from build123d import *

# Parameters (mm, degrees)
SKETCH1_W           = 50
SKETCH1_H           = 50
SKETCH1_W_2         = 46
SKETCH1_H_2         = 46
BOSS_EXTRUDE1_DEPTH = 10
SKETCH2_W           = 63.639610306
SKETCH2_H           = 63.639610306
SKETCH2_R           = 1.5
BOSS_EXTRUDE2_DEPTH = 3
FILLET2_R           = 5
FILLET3_R           = 2
CHAMFER2_SIZE       = 1


with BuildPart() as part:
    # Sketch1 → Boss-Extrude1 (new body)
    with BuildSketch(Plane(origin=(0, 0, 0), x_dir=(1, 0, 0), z_dir=(0, 1, 0))):
        Rectangle(SKETCH1_W, SKETCH1_H)
        Rectangle(SKETCH1_W_2, SKETCH1_H_2, mode=Mode.SUBTRACT)
    extrude(amount=BOSS_EXTRUDE1_DEPTH)

    # Sketch2 → Boss-Extrude2 (add)
    with BuildSketch(Plane(origin=(0, 10, 0), x_dir=(1, 0, 0), z_dir=(0, 1, 0))):
        Rectangle(SKETCH2_W, SKETCH2_H)
        with Locations(Location((-27.577164466, 27.577164466, 0), (0, 0, 270))):
            Circle(SKETCH2_R, mode=Mode.SUBTRACT)
        with Locations(Location((27.577164466, 27.577164466, 0), (0, 0, 270))):
            Circle(SKETCH2_R, mode=Mode.SUBTRACT)
        with Locations(Location((-27.577164466, -27.577164466, 0), (0, 0, 270))):
            Circle(SKETCH2_R, mode=Mode.SUBTRACT)
        with Locations(Location((27.577164466, -27.577164466, 0), (0, 0, 270))):
            Circle(SKETCH2_R, mode=Mode.SUBTRACT)
        with BuildLine():
            Line((-5, -23), (5, -23))
            Line((5, -23), (5, -18))
            ThreePointArc((5, -18), (0, -13), (-5, -18))
            Line((-5, -18), (-5, -23))
        make_face(mode=Mode.SUBTRACT)
    extrude(amount=BOSS_EXTRUDE2_DEPTH)

    # Fillet2
    fillet2_edges = [part.edges().sort_by_distance(p)[0] for p in [
        (-25, 5, -25),
        (25, 5, -25),
        (25, 5, 25),
        (-25, 5, 25),
    ]]
    fillet(fillet2_edges, radius=FILLET2_R)

    # Fillet3
    fillet3_edges = [part.edges().sort_by_distance(p)[0] for p in [
        (31.819805153, 11.5, 31.819805153),
        (31.819805153, 11.5, -31.819805153),
        (-31.819805153, 11.5, -31.819805153),
        (-31.819805153, 11.5, 31.819805153),
    ]]
    fillet(fillet3_edges, radius=FILLET3_R)

    # Chamfer2
    chamfer2_edges = [part.edges().sort_by_distance(p)[0] for p in [
        (31.234018716, 13, -31.234018716),
        (0, 13, -31.819805153),
        (31.819805153, 13, 0),
        (-31.819805153, 13, 0),
        (0, 13, 31.819805153),
        (31.234018716, 13, 31.234018716),
        (-31.234018716, 13, 31.234018716),
        (-31.234018716, 13, -31.234018716),
    ]]
    chamfer(chamfer2_edges, length=CHAMFER2_SIZE)


solid = part.part
Read the model definition and answer for the solid it produces. Units are mm, in the model's axes. A direction names the side the tool comes from. Give positions to 0.01 mm unless a question says otherwise; leave off trailing zeros. Write each loop counter-clockwise with the first axis right and the second up, starting at its lowest first coordinate (ties: lowest second). Pieces come first, ordered by that corner, then holes. Notation, with made-up numbers: M 23.5,-6.75 L 43.5,-6.75 A35 cw 43.5,25.25 Z; hole C 73,53.25 d2. An arc over 180 degrees is marked long. One line per item, written item: value. Start each with the question number.
(1) Find section D-D (z = -14). Determine the outline of the cut face in (x, y), plus the area to 3 significant figures.
(2) A tool of negligible diameter and unlimited length cuts with its end or side. For faces 1 (the flat face through (23, 5, 0)), 2 (the cylindrical face through (-23, 5, -24)), 3 (the flat face through (0, 0, -24)), 4 (the cylindrical face through (24, 5, -23)), 5 (the flat face through (25, 5, 0)), from which of +Z, -Z, +X, -X, +Y, -Y can it reach the whole face along a straight path? Write none if from no direction.
(3) Find the intervals of material crossed by line 1 (X direction, y = 6, z = -1); line 2 (Y direction, x = 16, z = -7.5), in increasing order.
(4) Find section B-B (x = 4). Determine the outline of the cut face in (y, z), plus the area to 3 significant figures.
(5) Flat-ended cylindrical pins translate along their axes: pin 1 Ø3 at (x, z) = (9, -18.5) entering from -Y; pin 2 Ø3 at (y, z) = (6.5, -4) entering from -X; pin 3 Ø6 at (x, y) = (0.5, 6.5) entering from -Z; pin 4 Ø3.5 at (x, z) = (27.58, 27.58) entering from +Y. Find the tip coordinate at first contact, or state that the pin passes through.
(6) Find section A-A (z = 19). Determine the outline of the cut face in (x, y).
(7) Determine the mould class of faces 6 (the cylindrical face through (-28.15, 11.48, -26.19)), 7 (the cylindrical face through (0, 11, 13)), 8 (the flat face through (-25, 5, 0)), 9 (the flat face through (0, 5, -25)) for opening direction X: pulls with the +X half, pulls with the -X half, needs draft (parallel to the pull), parting line crosses it, or undercut.
(8) Find section C-C (y = 8.25). Determine the outline of the cut face in (x, z), plus the area to 3 significant figures.
Results below:
1. outline: M -31.82,10 L -25,10 L -25,0 L -23,0 L -23,10 L 23,10 L 23,0 L 25,0 L 25,10 L 31.82,10 L 31.82,12 L 30.82,13 L -30.82,13 L -31.82,12 Z
1. area: 230 mm^2
2. face 1: -Y
2. face 2: -Z, -X, -Y
2. face 3: +Z, -Z, +X, -X, -Y
2. face 4: -Z, +X, -Y
2. face 5: +Z, -Z, +X, -Y
3. line 1: x = -25 to -23, 23 to 25
3. line 2: y = 10 to 13
4. outline: M 0,-25 L 10,-25 L 10,-31.82 L 12,-31.82 L 13,-30.82 L 13,15 L 10,15 L 10,-23 L 0,-23 Z; M 0,23 L 13,23 L 13,30.82 L 12,31.82 L 10,31.82 L 10,25 L 0,25 Z
4. area: 206 mm^2
5. pin 1: stops at y = 10
5. pin 2: stops at x = -25
5. pin 3: stops at z = -25
5. pin 4: stops at y = 13
6. outline: M -31.82,10 L -25,10 L -25,0 L -23,0 L -23,10 L -5,10 L -5,13 L -30.82,13 L -31.82,12 Z; M 5,10 L 23,10 L 23,0 L 25,0 L 25,10 L 31.82,10 L 31.82,12 L 30.82,13 L 5,13 Z
7. face 6: undercut
7. face 7: undercut
7. face 8: pulls with the -X half
7. face 9: needs draft
8. outline: M -25,-20 A5 ccw -20,-25 L 20,-25 A5 ccw 25,-20 L 25,20 A5 ccw 20,25 L -20,25 A5 ccw -25,20 Z; hole M -23,-23 L 23,-23 L 23,23 L -23,23 Z
8. area: 363 mm^2
